```python
from build123d import *

# Parameters (mm, degrees)
BOSS_EXTRUDE1_DEPTH = 4.7625
SKETCH3_W           = 4.7625
SKETCH3_H           = 31.75
SKETCH3_H_2         = 29.028571429
CUT_EXTRUDE1_DEPTH  = 417.575850499


with BuildPart() as part:
    # Sketch1 → Boss-Extrude1 (new body)
    with BuildSketch(Plane(origin=(0, 0, 0), x_dir=(0, 0, -1), z_dir=(1, 0, 0))):
        Polygon((381, 152.4), (-385.7625, 152.4), (-385.7625, 108.176785714), (-381, 108.176785714), (-381, 63.953571429), (-385.7625, 63.953571429), (-385.7625, 19.730357143), (-381, 19.730357143), (-381, -24.492857143), (-385.7625, -24.492857143), (-385.7625, -68.716071429), (-381, -68.716071429), (-381, -112.939285714), (-385.7625, -112.939285714), (-385.7625, -152.4), (-326.414423077, -152.4), (-326.414423077, -157.1625), (-267.066346154, -157.1625), (-267.066346154, -152.4), (-207.718269231, -152.4), (-207.718269231, -157.1625), (-148.370192308, -157.1625), (-148.370192308, -152.4), (-89.022115385, -152.4), (-89.022115385, -157.1625), (-29.674038462, -157.1625), (-29.674038462, -152.4), (29.674038462, -152.4), (29.674038462, -157.1625), (89.022115385, -157.1625), (89.022115385, -152.4), (148.370192308, -152.4), (148.370192308, -157.1625), (207.718269231, -157.1625), (207.718269231, -152.4), (267.066346154, -152.4), (267.066346154, -157.1625), (326.414423077, -157.1625), (326.414423077, -152.4), (385.7625, -152.4), (385.7625, -112.939285714), (381, -112.939285714), (381, -68.716071429), (385.7625, -68.716071429), (385.7625, -24.492857143), (381, -24.492857143), (381, 19.730357143), (385.7625, 19.730357143), (385.7625, 63.953571429), (381, 63.953571429), (381, 108.176785714), (385.7625, 108.176785714), (385.7625, 152.4), align=None)
    extrude(amount=BOSS_EXTRUDE1_DEPTH)

    # Sketch3 → Cut-Extrude1 (cut, through all)
    with BuildSketch(Plane(origin=(4.7625, 0, 0), x_dir=(0, 0, -1), z_dir=(1, 0, 0))):
        with Locations((-121.44375, -104.775)):
            Rectangle(SKETCH3_W, SKETCH3_H)
        with Locations((-121.44375, -41.275)):
            Rectangle(SKETCH3_W, SKETCH3_H)
        with Locations((-121.44375, 22.225)):
            Rectangle(SKETCH3_W, SKETCH3_H)
        with Locations((-121.44375, 85.725)):
            Rectangle(SKETCH3_W, SKETCH3_H)
        with Locations((-132.55625, 61.685714285)):
            Rectangle(SKETCH3_W, SKETCH3_H_2)
        with Locations((-132.55625, 3.628571428)):
            Rectangle(SKETCH3_W, SKETCH3_H_2)
        with Locations((-132.55625, -54.428571428)):
            Rectangle(SKETCH3_W, SKETCH3_H_2)
        with Locations((-132.55625, -112.485714286)):
            Rectangle(SKETCH3_W, SKETCH3_H_2)
        with Locations((132.55625, 85.725)):
            Rectangle(SKETCH3_W, SKETCH3_H)
        with Locations((121.44375, 61.685714285)):
            Rectangle(SKETCH3_W, SKETCH3_H_2)
        with Locations((132.55625, 22.225)):
            Rectangle(SKETCH3_W, SKETCH3_H)
        with Locations((121.44375, 3.628571428)):
            Rectangle(SKETCH3_W, SKETCH3_H_2)
        with Locations((132.55625, -41.275)):
            Rectangle(SKETCH3_W, SKETCH3_H)
        with Locations((121.44375, -54.428571428)):
            Rectangle(SKETCH3_W, SKETCH3_H_2)
        with Locations((132.55625, -104.775)):
            Rectangle(SKETCH3_W, SKETCH3_H)
        with Locations((121.44375, -112.485714286)):
            Rectangle(SKETCH3_W, SKETCH3_H_2)
    extrude(amount=-CUT_EXTRUDE1_DEPTH, mode=Mode.SUBTRACT)


solid = part.part
```
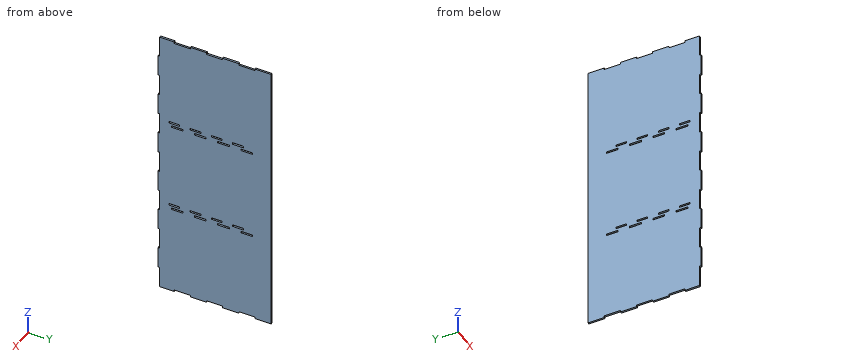
Work out the finished part from the listing and answer in its coordinate system (mm). Coordinates: 2 decimals unless noted, no trailing zeros.
1) Flat-ended cylindrical pins translate along their axes: pin 1 (1.4 mm diameter, centred on x = 2, z = -120.5, fed in from -Y); pin 2 (1.4 mm diameter, centred on x = 3, y = -1.5, fed in from +Z). Find the tip coordinate at first contact, or state that the pin passes through.
Results:
pin 1: stops at y = -152.4
pin 2: stops at z = 381
2) Section A-A (x = 1) is taken. Give the number of separate pieces and of enclosed holes in the cut face, plus the area to 3 significant figures.
Results:
separate pieces: 1
enclosed holes: 16
area: 233,000 mm2
3) Consider probe 1 along Z at (x, y) = (3.65, 24) (1 decimal); probe 2 along Z at (x, y) = (2.3, -121) (1 decimal); probe 3 along Z at (x, y) = (1.25, -56) (1 decimal). Determine where each line is inside the solid, lowest interval first.
Results:
probe 1: z = -385.8 to -134.9, -130.2 to 119.1, 123.8 to 385.8
probe 2: z = -385.8 to -123.8, -119.1 to 130.2, 134.9 to 385.8
probe 3: z = -385.8 to -134.9, -130.2 to -123.8, -119.1 to 119.1, 123.8 to 130.2, 134.9 to 385.8
